Design review of the part built by this model. Coordinates are the model's own, in mm. Face numbers are marked on the shaded views. A direction names the side the tool comes from. Give positions to 0.01 mm unless a question says otherwise; leave off trailing zeros. Loops run counter-clockwise (first coordinate to the right, second up) from the corner with the lowest first, then second, coordinate; pieces in that order, holes last.
Autodesk Inventor part; units mm, degrees
ref_plane "Work Plane1" through (0, 75, 0) normal (0, 1, 0) x (1, 0, 0)
ref_plane "YZ Plane" through (0, 0, 0) normal (1, 0, 0) x (0, 1, 0)
ref_plane "XZ Plane" through (0, 0, 0) normal (0, 1, 0) x (-1, 0, 0)
sketch "Sketch1" plane through (0, 0, 0) normal (0, 1, 0) x (-1, 0, 0)
  arc A0 (-25, 0) -> (25, 0) centre (0, 0) ccw
  arc A1 (-29.5804, -5) -> (29.5804, -5) centre (0, 0) ccw
  line L0 (25, 0) -> (55, 0)
  line L1 (55, 0) -> (55, -5)
  line L2 (55, -5) -> (29.5804, -5)
  line L3 (-25, 0) -> (-45, 0)
  line L4 (-45, -5) -> (-29.5804, -5)
  line L5 (0, 0) -> (12.5, 0) construction
  line L6 (12.5, -300) -> (0, -300) construction
  line L7 (0, -185) -> (0, 0) construction
  line L8 (0, 0) -> (-12.5, 0) construction
  line L9 (-12.5, -300) -> (0, -300) construction
  line L10 (0, 0) -> (0, -150) construction
  line L11 (-40, -150) -> (40, -150)
  line L12 (40, -160) -> (40, -210)
  line L13 (-30, -210) -> (-40, -210) construction
  line L14 (-40, -210) -> (-40, -160)
  line L15 (-40, -150) -> (40, -210) construction
  line L16 (40, -150) -> (-40, -210) construction
  line L17 (40, -150) -> (50, -150)
  line L18 (50, -150) -> (50, -210)
  line L19 (50, -210) -> (40, -210)
  line L20 (-40, -150) -> (-50, -150)
  line L21 (-50, -150) -> (-50, -210)
  line L22 (-50, -210) -> (-40, -210)
  line L23 (12.5, -150) -> (12.5, -160) construction
  line L24 (12.5, -150) -> (12.5, -160)
  line L25 (40, -160) -> (12.5, -160)
  line L26 (-12.5, -160) -> (-40, -160)
  line L27 (0, -160) -> (20, -160) construction
  line L28 (20, -160) -> (20, -170)
  line L29 (20, -170) -> (30, -170)
  line L30 (30, -170) -> (30, -185)
  line L31 (30, -185) -> (0, -185)
  line L32 (0, -160) -> (-20, -160) construction
  line L33 (-20, -160) -> (-20, -170)
  line L34 (-20, -170) -> (-30, -170)
  line L35 (-30, -170) -> (-30, -185)
  line L36 (-30, -185) -> (0, -185)
  line L37 (-25, 0) -> (-55, 0)
  line L38 (-55, -5) -> (-29.5804, -5)
  line L39 (-55, 0) -> (-55, -5)
  line L40 (12.5, -27.2718) -> (12.5, -150)
  line L41 (-12.5, -27.2718) -> (-12.5, -150)
  point P0 (0, -180)
  dimension "d0" = 50
  dimension "d1" = 60
  dimension "d2" = 30
  dimension "d3" = 5
  dimension "d5" = 5
  dimension "d6" = 12.5
  dimension "d7" = 300
  dimension "d8" = 150
  dimension "d9" = 80
  dimension "d10" = 60
  dimension "d11" = 10
  dimension "d12" = 10
  dimension "d13" = 20
  dimension "d14" = 10
  dimension "d15" = 10
  dimension "d16" = 15
extrude "Extrusion1" add sketch "Sketch1" along normal blind 150 contours A0 L0 L1 L2 A1 L4 L38 L39 L37 L3
ref_plane "Work Plane1" through (0, 75, 0) normal (0, 1, 0) x (1, 0, 0)
sketch "Sketch3" plane through (0, 75, 0) normal (0, 1, 0) x (1, 0, 0)
  line L0 (25, 0) -> (55, 0)
  line L1 (-25, 0) -> (-45, 0)
  line L2 (0, 0) -> (12.5, 0) construction
  line L3 (0, 0) -> (-12.5, 0) construction
  line L4 (-25, 0) -> (-55, 0)
  arc A0 (25, 0) -> (-25, 0) centre (0, 0) ccw
  arc A1 (29.5804, 5) -> (-29.5804, 5) centre (0, 0) ccw
  line L5 (55, 0) -> (55, 5)
  line L6 (55, 5) -> (29.5804, 5)
  line L7 (-45, 5) -> (-29.5804, 5)
  line L8 (0, 185) -> (0, 0) construction
  line L9 (0, 0) -> (0, 150) construction
  line L10 (-40, 150) -> (40, 210) construction
  line L11 (40, 150) -> (-40, 210) construction
  line L12 (40, 150) -> (50, 150)
  line L13 (50, 150) -> (50, 200)
  line L14 (-50, 150) -> (-50, 200)
  line L15 (-40, 150) -> (-50, 150)
  line L16 (0, 160) -> (12.5, 160) construction
  line L17 (20, 160) -> (20, 170)
  line L18 (20, 170) -> (30, 170)
  line L19 (30, 170) -> (30, 185)
  line L20 (30, 185) -> (0, 185)
  line L21 (0, 160) -> (-12.5, 160) construction
  line L22 (-20, 160) -> (-20, 170)
  line L23 (-20, 170) -> (-30, 170)
  line L24 (-30, 170) -> (-30, 185)
  line L25 (-30, 185) -> (0, 185)
  line L26 (-55, 5) -> (-29.5804, 5)
  line L27 (12.5, 27.2718) -> (12.5, 130)
  line L28 (-12.5, 27.2718) -> (-12.5, 130)
  line L29 (-40, 150) -> (-20, 150)
  line L30 (20, 150) -> (40, 150)
  line L31 (-70, 200) -> (-70, 140)
  line L32 (50, 150) -> (50, 200)
  line L33 (-50, 200) -> (-50, 150)
  line L34 (-50, 150) -> (50, 210) construction
  line L35 (50, 150) -> (-50, 210) construction
  line L36 (20, 160) -> (20, 150)
  line L37 (-20, 160) -> (-20, 150)
  line L38 (-50, 150) -> (-20, 150)
  line L39 (20, 150) -> (50, 150)
  line L40 (70, 200) -> (70, 140)
  line L41 (-50, 150) -> (50, 150)
  line L42 (50, 150) -> (50, 200)
  line L43 (-50, 200) -> (-50, 150)
  line L44 (-70, 140) -> (-70, 130)
  line L45 (-70, 130) -> (-12.5, 130)
  line L46 (12.5, 130) -> (70, 130)
  line L47 (70, 130) -> (70, 140)
  line L48 (-50, 200) -> (50, 200)
  line L49 (70, 200) -> (70, 220)
  line L50 (70, 220) -> (-70, 220)
  line L51 (-70, 220) -> (-70, 200)
  point P0 (-45, -5)
  point P1 (0, 180)
  dimension "d21" = 30
  dimension "d62" = 50
  dimension "d63" = 10
  dimension "d65" = 20
extrude "Extrusion2" add sketch "Sketch3" along normal mid plane 50 contours A1 L28 L45 L44 L31 L51 L50 L49 L40 L47 L46 L27 | L41 L37 L22 L23 L24 L25 L20 L19 L18 L17 L36
sketch "Sketch5" plane through (-50, 50, -150) normal (1, 0, 0) x (0, 0, 1)
  line L0 (-35, 0) -> (-35, -50) construction
  circle A0 centre (-35, -25) radius 10
  point P0 (150, 50)
  dimension "d38" = 20
extrude "Extrusion4" cut sketch "Sketch5" against normal blind 20
sketch "Sketch6" plane through (55, 0, -5) normal (0, 0, -1) x (-1, 0, 0)
  line L0 (30, 0) -> (0, 0)
  line L1 (15, 0) -> (15, 50) construction
  line L2 (15, 50) -> (15, 100) construction
  circle A0 centre (15, 100) radius 5
  circle A1 centre (15, 50) radius 5
  point P0 (55, 0)
  dimension "d43" = 50
  dimension "d44" = 50
  dimension "d45" = 10
  dimension "d46" = 10
extrude "Extrusion5" cut sketch "Sketch6" against normal blind 10
sketch "Sketch7" plane through (-29.5804, 0, -5) normal (0, 0, -1) x (-1, 0, 0)
  line L0 (25.4196, 0) -> (-4.5804, 0)
  line L1 (10.4196, 50) -> (10.4196, 100) construction
  line L2 (10.4196, 0) -> (10.4196, 50) construction
  line L3 (10.4196, 50) -> (10.4196, 100)
  circle A0 centre (10.4196, 100) radius 5
  circle A1 centre (10.4196, 50) radius 5
  point P0 (-29.5804, 0)
  dimension "d49" = 50
  dimension "d50" = 50
  dimension "d51" = 10
  dimension "d52" = 10
extrude "Extrusion6" cut sketch "Sketch7" against normal blind 10
fillet "Fillet2" radius 3 4 edges at (70, 75, -130) (12.5, 75, -130) (-12.5, 75, -130) (-70, 75, -130)
sketch "Sketch8" plane through (70, 50, -220) normal (1, 0, 0) x (0, 0, -1)
  line L0 (-35, 0) -> (-35, 50)
  circle A0 centre (-35, 25) radius 10
  point P0 (-220, -50)
  dimension "d66" = 20
extrude "Extrusion7" cut sketch "Sketch8" against normal blind 20
thread "Thread1"
properties part number "Clamp jaw"
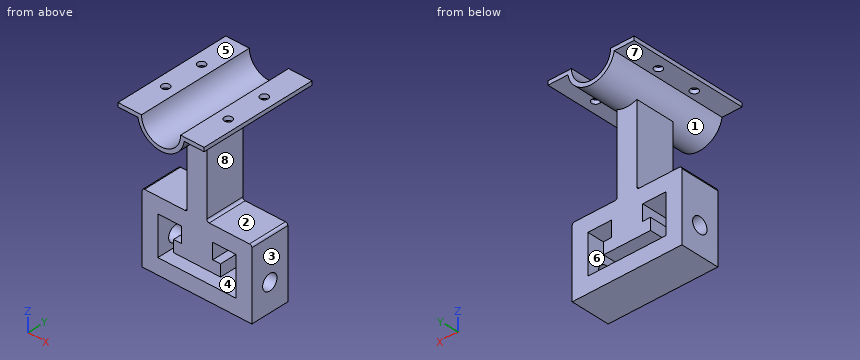
Q1. Draft analysis for pull direction X (two halves, no side actions). For the marked faces 1, 2, 3 and 4, state which applies: pulls with the +X half, pulls with the -X half, needs draft (parallel to the pull), parting line crosses it, or undercut.
Results:
face 1: parting line crosses it
face 2: needs draft
face 3: pulls with the +X half
face 4: undercut
Q2. Tool access review of the marked faces 5, 6, 7 and 8: name each direction out of +Z, -Z, +X, -X, +Y, -Y from which nothing blocks a thin tool from reaching the whole face with its end or side.
Results:
face 5: +Z, +X, -X, +Y, -Y
face 6: +Y, -Y
face 7: -X, +Y, -Y
face 8: +X, +Y, -Y
Q3. Take a section at C-C (x = -4.5). Give the boundary of the cut face in (y, z).
Results:
outline: (0, -29.66) - (50, -29.66) - (50, -185) - (100, -185) - (100, -29.66) - (150, -29.66) - (150, -24.59) - (0, -24.59) - close; (50, -220) - (100, -220) - (100, -200) - (50, -200) - close
Q4. Take a section at A-A (x = -40). Give the boundary of the cut face in (y, z).
Results:
outline: (0, -5) - (45, -5) - (45, 0) - (0, 0) - close; (50, -220) - (100, -220) - (100, -200) - (50, -200) - close; (50, -150) - (100, -150) - (100, -130) - (50, -130) - close; (55, -5) - (95, -5) - (95, 0) - (55, 0) - close; (105, -5) - (150, -5) - (150, 0) - (105, 0) - close
Q5. Take a section at D-D (y = 97.5). Give the number of separate pieces and of enclosed holes in the cut face, plus the area to 3 significant figures.
Results:
separate pieces: 3
enclosed holes: 1
area: 12,400 mm2
Q6. Wall thickness on line 1 (Y direction, x = 40, z = -1); line 2 (X direction, y = 84, z = -158); line 3 (Y direction, x = 60.25, z = -185): over which ranges is each line inside the solid? List them lowest first.
Results:
line 1: y = 0 to 45, 55 to 95, 105 to 150
line 2: x = -70 to -50, -20 to 20, 50 to 70
line 3: y = 50 to 65, 85 to 100
Q7. Insertion check: pin 1 (6 mm diameter, centred on x = -1.5, y = 43, fed in from -Z); pin 2 (10 mm diameter, centred on x = 40, y = 130.5, fed in from -Z); pin 3 (6 mm diameter, centred on y = 80.5, z = -124, fed in from +X); pin 4 (15 mm diameter, centred on x = -36.5, y = 75, fed in from +Z). Each pin has a flat end and moves straight along its axis. Give the tip position at first contact, or say it passes through.
Results:
pin 1: stops at z = -30
pin 2: stops at z = -5
pin 3: stops at x = 12.5
pin 4: stops at z = 0
